from build123d import *

# Parameters (mm, degrees)
SKETCH2_W               = 25
SKETCH2_H               = 10
BOSS_EXTRUDE1_DEPTH     = 5
FILLET1_RADIUS          = 5
FILLET1_LENGTH          = 5
SKETCH3_W               = 4
SKETCH3_H               = 10
BOSS_EXTRUDE2_DEPTH     = 17
SKETCH12_R              = 2.5
CUT_EXTRUDE3_DEPTH      = 5
CUT_EXTRUDE4_DEPTH      = 3
SKETCH14_R              = 3.5
CUT_EXTRUDE5_DEPTH      = 2
SKETCH15_W              = 10
SKETCH15_H              = 15.5
BOSS_EXTRUDE3_DEPTH     = 16
SKETCH16_W              = 16
SKETCH16_H              = 2
CUT_EXTRUDE6_DEPTH      = 31
CUT_EXTRUDE9_DEPTH      = 54.030651514
CUT_EXTRUDE9_DEPTH_BACK = 6
SKETCH18_W              = 13
SKETCH18_H              = 25
RIB1_REACH              = 54.662
SKETCH20_WALL_W         = 124.593227798
SKETCH20_WALL_H         = 3
RIB2_REACH              = 54.662
SKETCH21_WALL_W         = 124.593227798
SKETCH21_WALL_H         = 3
SKETCH22_R              = 0.8
CUT_EXTRUDE10_DEPTH     = 6
BOSS_EXTRUDE4_DEPTH     = 15.5
SKETCH39_W              = 3
SKETCH39_H              = 4.8
BOSS_EXTRUDE5_DEPTH     = 17
SKETCH42_W              = 4
SKETCH42_H              = 4.8
BOSS_EXTRUDE6_DEPTH     = 10.5
SKETCH43_R              = 2.4
BOSS_EXTRUDE7_DEPTH     = 2.5


with BuildPart() as part:
    # Sketch2 → Boss-Extrude1 (new body)
    with BuildSketch(Plane(origin=(0, 0, 0), x_dir=(1, 0, 0), z_dir=(0, 1, 0))):
        Rectangle(SKETCH2_W, SKETCH2_H)
    extrude(amount=BOSS_EXTRUDE1_DEPTH)

    # Fillet1: full round fillet: the end face becomes a half cylinder, R = half its width
    fillet1_face = Plane((12.5, 2.5, 0), x_dir=(0, -1, 0), z_dir=(1, 0, 0))  # on the end face: x along it, z out of the body
    fillet1_slab = fillet1_face.offset(-FILLET1_RADIUS / 2) * Box(FILLET1_LENGTH, 2 * FILLET1_RADIUS, FILLET1_RADIUS, mode=Mode.PRIVATE)  # the body's end, R deep
    fillet1_round = Plane((7.5, 2.5, 0), x_dir=(1, 0, 0), z_dir=(0, -1, 0)) * Cylinder(FILLET1_RADIUS, FILLET1_LENGTH, mode=Mode.PRIVATE)  # its axis R under the face
    add(fillet1_slab - fillet1_round, mode=Mode.SUBTRACT)

    # Sketch3 → Boss-Extrude2 (add)
    with BuildSketch(Plane(origin=(0, 5, 0), x_dir=(1, 0, 0), z_dir=(0, 1, 0))):
        with Locations((-10.5, 0)):
            Rectangle(SKETCH3_W, SKETCH3_H)
    extrude(amount=BOSS_EXTRUDE2_DEPTH)

    # Mirror1: part across plane


with BuildPart() as part_1:
    add(part.part)
    add(part.part.mirror(Plane.ZX.offset(22)))

    # Sketch12 → Cut-Extrude3 (cut)
    with BuildSketch(Plane(origin=(0, 44, 0), x_dir=(1, 0, 0), z_dir=(0, 1, 0))):
        with Locations(Location((7.5, 0, 0), (0, 0, 270))):
            Circle(SKETCH12_R)
    extrude(amount=-CUT_EXTRUDE3_DEPTH, mode=Mode.SUBTRACT)

    # Sketch13 → Cut-Extrude4 (cut)
    with BuildSketch(Plane.XZ):
        with BuildLine():
            Line((7.195652174, 3.486742377), (-8.782608696, 2.092045426))
            ThreePointArc((-8.782608696, 2.092045426), (-10.7, 0), (-8.782608696, -2.092045426))
            Line((-8.782608696, -2.092045426), (7.195652174, -3.486742377))
            ThreePointArc((7.195652174, -3.486742377), (11, 0), (7.195652174, 3.486742377))
        make_face()
    extrude(amount=-CUT_EXTRUDE4_DEPTH, mode=Mode.SUBTRACT)

    # Sketch14 → Cut-Extrude5 (cut)
    with BuildSketch(Plane.XZ.offset(-3)):
        with Locations(Location((7.5, 0, 0), (0, 0, 270))):
            Circle(SKETCH14_R)
    extrude(amount=-CUT_EXTRUDE5_DEPTH, mode=Mode.SUBTRACT)

    # Sketch15 → Boss-Extrude3 (add)
    with BuildSketch(Plane.ZY.offset(12.5)):
        with Locations((0, 14.25)):
            Rectangle(SKETCH15_W, SKETCH15_H)
        with Locations((0, 29.75)):
            Rectangle(SKETCH15_W, SKETCH15_H)
    extrude(amount=BOSS_EXTRUDE3_DEPTH)

    # Sketch16 → Cut-Extrude6 (cut)
    with BuildSketch(Plane.XZ.offset(-6.5)):
        with Locations((-20.5, 4)):
            Rectangle(SKETCH16_W, SKETCH16_H)
        with Locations((-20.5, -4)):
            Rectangle(SKETCH16_W, SKETCH16_H)
    extrude(amount=-CUT_EXTRUDE6_DEPTH, mode=Mode.SUBTRACT)

    # Sketch18 → Cut-Extrude9 (cut, two sides: drawn at the far end of the back side and taken through both)
    with BuildSketch(Plane(origin=(0, 0, -3), x_dir=(-1, 0, 0), z_dir=(0, 0, -1)).offset(-CUT_EXTRUDE9_DEPTH_BACK)):
        with Locations((19, 22)):
            Rectangle(SKETCH18_W, SKETCH18_H)
    extrude(amount=CUT_EXTRUDE9_DEPTH + CUT_EXTRUDE9_DEPTH_BACK, mode=Mode.SUBTRACT)

    # Sketch20 wall → Rib1 (add, up to next)
    with BuildSketch(Plane(origin=(-20.5, 40.75, 0), x_dir=(0.926466577122, 0.376377046956, 0), z_dir=(-0.376377046956, 0.926466577122, 0)), mode=Mode.PRIVATE) as rib1_sk1:
        Rectangle(SKETCH20_WALL_W, SKETCH20_WALL_H)
    rib1_tool1 = extrude(rib1_sk1.sketch, amount=-RIB1_REACH, mode=Mode.PRIVATE) - part_1.part
    add(rib1_tool1.solids().sort_by_distance((-20.5, 40.75, 0))[0])

    # Sketch21 wall → Rib2 (add, up to next)
    with BuildSketch(Plane(origin=(-20.5, 3.25, 0), x_dir=(0.926466577122, -0.376377046956, 0), z_dir=(0.376377046956, 0.926466577122, 0)), mode=Mode.PRIVATE) as rib2_sk1:
        Rectangle(SKETCH21_WALL_W, SKETCH21_WALL_H)
    rib2_tool1 = extrude(rib2_sk1.sketch, amount=RIB2_REACH, mode=Mode.PRIVATE) - part_1.part
    add(rib2_tool1.solids().sort_by_distance((-20.5, 3.25, 0))[0])

    # Sketch22 → Cut-Extrude10 (cut)
    with BuildSketch(Plane.XY.offset(3)):
        with Locations((-19, 36)):
            Circle(SKETCH22_R)
        with Locations(Location((-19, 8, 0), (0, 0, 180))):
            Circle(SKETCH22_R)
    extrude(amount=-CUT_EXTRUDE10_DEPTH, mode=Mode.SUBTRACT)

    # Sketch38 → Boss-Extrude4 (add)
    with BuildSketch(Plane.XY.offset(3)):
        Polygon((-25.5, 27.3), (-25.5, 24.9), (-28.5, 24.9), (-28.5, 29.7), (-25.5, 29.7), align=None)
    extrude(amount=BOSS_EXTRUDE4_DEPTH)

    # Sketch39 → Boss-Extrude5 (add)
    with BuildSketch(Plane(origin=(-25.5, 0, 0), x_dir=(0, 0, -1), z_dir=(1, 0, 0))):
        with Locations((-17, 27.3)):
            Rectangle(SKETCH39_W, SKETCH39_H)
    extrude(amount=BOSS_EXTRUDE5_DEPTH)

    # Sketch42 → Boss-Extrude6 (add)
    with BuildSketch(Plane(origin=(0, 0, 15.5), x_dir=(-1, 0, 0), z_dir=(0, 0, -1))):
        with Locations((10.5, 27.3)):
            Rectangle(SKETCH42_W, SKETCH42_H)
    extrude(amount=BOSS_EXTRUDE6_DEPTH)

    # Sketch43 → Boss-Extrude7 (add)
    with BuildSketch(Plane.XY.offset(18.5)):
        with Locations(Location((-19, 27.3, 0), (0, 0, 270))):
            Circle(SKETCH43_R)
    extrude(amount=BOSS_EXTRUDE7_DEPTH)


solid = part_1.part
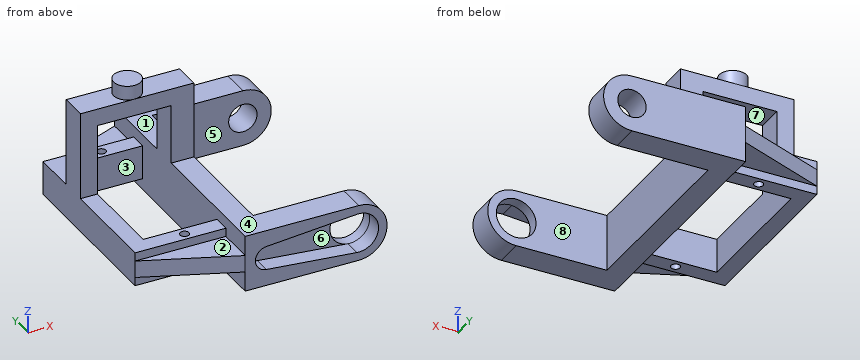
Model file for the job. Use its own axes, mm. Face numbers are marked on the shaded views. A direction names the side the tool comes from. Round coordinates to 2 decimals unless told otherwise and drop trailing zeros. Order: outer loops, then holes, each group sorted by start corner. A loop starts at its lowest first (then second) coordinate and runs counter-clockwise, first axis right, second up. Notation, with made-up numbers: M 74.5,-33 L 110.5,-33 A18 cw 110.5,-26 Z; hole C -35.75,11.5 d4. An arc over 180 degrees is marked long. Write each question's results on one line, items separated by ' | '. Start each with the question number.
(1) Which spindle directions (+Z, -Z, +X, -X, +Y, -Y) get a long thin tool onto all of the face, cutting with end or side? Do the marked faces 1, 2, 3, 4 and 5. Say none if no direction does.
(2) Saw through at B-B, the plane y = 12. Give the cut face in (x, z).
(3) Drop flat-ended pins along their axis: pin 1 (5.5 mm diameter, centred on y = 24.5, z = 2, fed in from +X); pin 2 (17.5 mm diameter, centred on x = -23, y = 15, fed in from +Z); pin 3 (6 mm diameter, centred on x = -16.5, z = 1.5, fed in from +Y); pin 4 (8 mm diameter, centred on x = 3.5, z = 2, fed in from -Y). Give the stop position or say it passes through.
(4) Saw through at A-A, the plane z = 0. Give the cut face in (x, y).
(5) Saw through at C-C, the plane z = 12. Give the cut face in (x, y), then the cut area to 3 significant figures.
(6) Two-plate mould, pull along Z, no slides. Class the marked faces 6, 7 and 8: pulls with the +Z half, pulls with the -Z half, needs draft (parallel to the pull), parting line crosses it, or undercut.
(7) Saw through at D-D, the plane x = 9. Give the cut face in (y, z), then the cut area to 3 significant figures.
(8) Probe probe 1 along Y at (x, z) = (-3, -1); probe 2 along Y at (x, z) = (-19, 1.7); probe 3 along Z at (x, y) = (7.5, 3.75). List the from-to ranges inside material, lowest first. Write a range as from..to.
Established:
1) face 1: +Z, +X, -X, +Y | face 2: +Z, -X, -Y | face 3: +Z, -Z | face 4: +Z, +X, -X, -Y | face 5: +Z, -Z, +X
2) outline: M -28.5,-3 L -25.5,-3 L -25.5,3 L -28.5,3 Z; M -12.5,-5 L -8.5,-5 L -8.5,5 L -12.5,5 Z
3) pin 1: stops at x = -8.5 | pin 2: stops at z = 3 | pin 3: stops at y = 43.59 | pin 4: stops at y = 0
4) outline: M -28.5,6.5 L -12.5,0 L -10.7,0 L -10.7,3 L 4,3 L 4,5 L -8.5,5 L -8.5,39 L 5,39 L 5,44 L -12.5,44 L -28.5,37.5 Z; M 10,39 L 12.5,39 L 12.5,44 L 10,44 Z; M 11,0 L 12.5,0 L 12.5,5 L 11,5 Z; hole M -25.5,9.5 L -12.5,9.5 L -12.5,34.5 L -25.5,34.5 Z; hole C -19,8 d1.6; hole C -19,36 d1.6
5) outline: M -28.5,24.9 L -25.5,24.9 L -25.5,29.7 L -28.5,29.7 Z; M -12.5,24.9 L -8.5,24.9 L -8.5,29.7 L -12.5,29.7 Z | area: 33.6 mm^2
6) face 6: undercut | face 7: pulls with the -Z half | face 8: needs draft
7) outline: M 0,-4.77 L 5,-4.77 L 5,-3.16 L 0,-3.16 Z; M 0,3.16 L 5,3.16 L 5,4.77 L 0,4.77 Z; M 39,-4.77 L 44,-4.77 L 44,-2 L 39,-2 Z; M 39,2 L 44,2 L 44,4.77 L 39,4.77 Z | area: 43.8 mm^2
8) probe 1: y = 3..5, 39..44 | probe 2: y = 6.5..7.2, 8.8..9.5, 34.5..35.2, 36.8..37.5 | probe 3: z = -5..-3.5, 3.5..5
